For this review, use the dimensioned drawing (mm, ordinates from the lowest corner) and the shaded views. Coordinates: 2 decimals unless noted, no trailing zeros. Loops run counter-clockwise (first coordinate to the right, second up) from the corner with the lowest first, then second, coordinate; pieces in that order, holes last. Notation, with made-up numbers: (55.25, 3) - (102.25, 3) arc R23 ccw to (102.25, 19) - close; hole circle Ø8 at (85, -7.75). An arc over 180 degrees is marked (long way). Answer in a Markdown table with one row per item. Add a question column.
(1) Clearance check with a flat-ended pin moving along its axis: pin 1 (1.1 mm diameter, centred on x = 2.5, y = 6.5, fed in from +Z) (1 decimal). State where the tip first meets the part, or that it passes through.
(2) We need section C-C, the plane z = 14.5. Write out the cut boundary in (x, y).
(3) We need section B-B, the plane x = 4.25. Write out the cut boundary in (y, z) (1 decimal), plus the area to 3 significant figures.
(4) We need section D-D, the plane y = 9.25. Write out the cut boundary in (x, z) (1 decimal), plus the area to 3 significant figures.
(5) To check wall thickness, follow L1, parallel to Y at x = 3.25, z = 15; L2, parallel to X at y = 6.25, z = 15.5 (1 decimal); L3, parallel to Y at x = 4.75, z = 17 (1 decimal). State the ranges of each line that lie inside material, in increasing order. Write a range as [from, to].
(6) The part is to be moulded in two halves that separate along X. For the marked faces 1, 2 and 3, say which applies: released by +X, released by -X, zero draft, split by the parting line, or undercut.
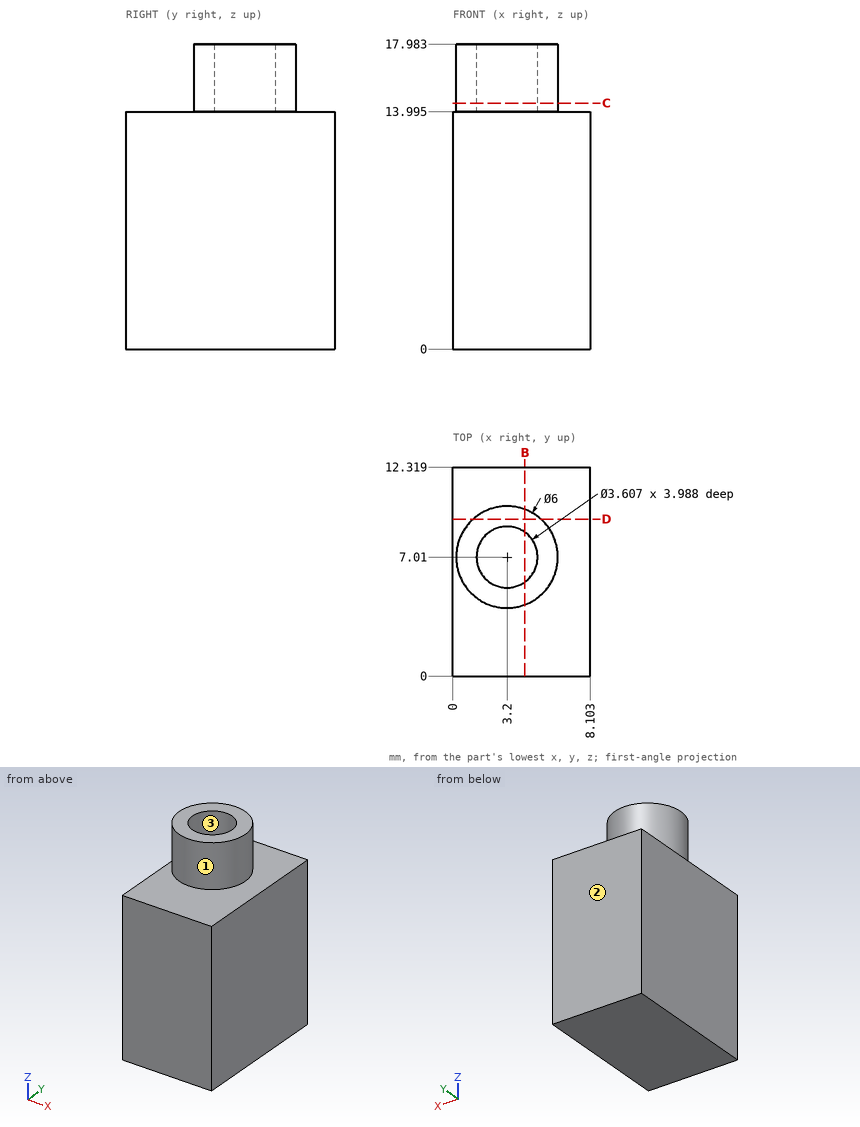
Responses:
| question | item | result |
|---|---|---|
| 1 | pin 1 | stops at z = 14 |
| 2 | outline | circle Ø6 at (3.2, 7.01); hole circle Ø3.61 at (3.2, 7.01) |
| 3 | outline | (0, 0) - (12.3, 0) - (12.3, 14) - (9.8, 14) - (9.8, 18) - (8.5, 18) - (8.5, 14) - (5.5, 14) - (5.5, 18) - (4.2, 18) - (4.2, 14) - (0, 14) - close |
| 3 | area | 183 mm2 |
| 4 | outline | (0, 0) - (8.1, 0) - (8.1, 14) - (5.2, 14) - (5.2, 18) - (1.2, 18) - (1.2, 14) - (0, 14) - close |
| 4 | area | 129 mm2 |
| 5 | L1 | y = [4.01, 5.21], [8.81, 10.01] |
| 5 | L2 | x = [0.3, 1.6], [4.8, 6.1] |
| 5 | L3 | y = [4.4, 6.1], [7.9, 9.6] |
| 6 | face 1 | split by the parting line |
| 6 | face 2 | zero draft |
| 6 | face 3 | undercut |
